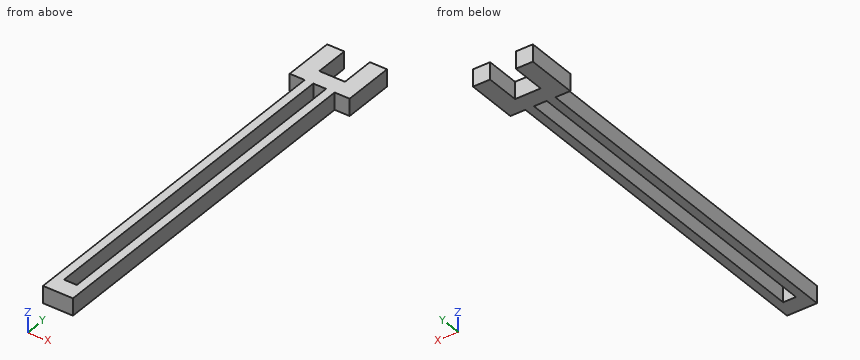
from build123d import *

# Parameters (mm, degrees)
F0_W     = 44.45
F0_H     = 25.4
F1_DEPTH = 533.4
F2_W     = 19.05
F2_H     = 508
F3_DEPTH = 25.4
F4_W     = 88.9
F4_H     = 25.4
F5_DEPTH = 76.2
F6_W     = 38.1
F6_H     = 50.8
F7_DEPTH = 25.4


with BuildPart() as f1:
    # F0 (on Front) → F1 (new body)
    with BuildSketch(Plane.XZ):
        Rectangle(F0_W, F0_H)
    extrude(amount=-F1_DEPTH)

    # F2 (on face) → F3 (cut)
    with BuildSketch(Plane.XY.offset(12.7)):
        with Locations((0, 279.4)):
            Rectangle(F2_W, F2_H)
    extrude(amount=-F3_DEPTH, mode=Mode.SUBTRACT)

    # F4 (on face) → F5 (join)
    with BuildSketch(Plane(origin=(0, 533.4, 0), x_dir=(-1, 0, 0), z_dir=(0, 1, 0))):
        Rectangle(F4_W, F4_H)
    extrude(amount=F5_DEPTH)

    # F6 (on face) → F7 (cut)
    with BuildSketch(Plane.XY.offset(12.7)):
        with Locations((0, 584.2)):
            Rectangle(F6_W, F6_H)
    extrude(amount=-F7_DEPTH, mode=Mode.SUBTRACT)


solid = f1.part
Geometry check sheet. Reference: the model listing, model coordinates, mm. Round coordinates to 2 decimals unless told otherwise and drop trailing zeros. Loops run counter-clockwise (first coordinate to the right, second up) from the corner with the lowest first, then second, coordinate; pieces in that order, holes last. Notation, with made-up numbers: (51.25, 37.25) - (60.25, 37.25) arc R18 cw to (60.25, 65.25) - close; hole circle Ø11 at (-31.75, 15.5). An arc over 180 degrees is marked (long way). One line per question, with ' | ' between items. Start each with the question number.
1. Cross-section at A-A on y = 262. Record the cut outline in (x, z) (3 decimals), then the cut area to 3 significant figures.
2. Cross-section at C-C on z = 2.25. Record the cut outline in (x, y) (3 decimals), then the cut area to 3 significant figures.
3. Scan lines: line 1 (X direction, y = 325, z = 8.75) (3 decimals); line 2 (X direction, y = 559, z = -11); line 3 (Y direction, x = 3, z = -3.75). Record each from-to range of solid material in increasing order. Write a range as [from, to].
4. Cross-section at D-D on x = 27.5. Record the cut outline in (y, z).
5. Cross-section at B-B on x = 4. Record the cut outline in (y, z), then the cut area to 3 significant figures.
6. Depth check by flat-ended pin: pin 1 (7.5 mm diameter, centred on y = 239.5, z = 5.5, fed in from +X) (3 decimals); pin 2 (11 mm diameter, centred on x = -29.5, z = -2.5, fed in from -Y); pin 3 (15 mm diameter, centred on x = 0, z = 2, fed in from +Y). Enter the tip coordinate at first touch or a pass-through.
Taken from the geometry:
1) outline: (-22.225, -12.7) - (-9.525, -12.7) - (-9.525, 12.7) - (-22.225, 12.7) - close; (9.525, -12.7) - (22.225, -12.7) - (22.225, 12.7) - (9.525, 12.7) - close | area: 645 mm²
2) outline: (-44.45, 533.4) - (-22.225, 533.4) - (-22.225, 0) - (22.225, 0) - (22.225, 533.4) - (44.45, 533.4) - (44.45, 609.6) - (19.05, 609.6) - (19.05, 558.8) - (-19.05, 558.8) - (-19.05, 609.6) - (-44.45, 609.6) - close; hole (-9.525, 25.4) - (9.525, 25.4) - (9.525, 533.4) - (-9.525, 533.4) - close | area: 18,900 mm²
3) line 1: [-22.225, -9.525], [9.525, 22.225] | line 2: [-44.45, -19.05], [19.05, 44.45] | line 3: [0, 25.4], [533.4, 558.8]
4) outline: (533.4, -12.7) - (609.6, -12.7) - (609.6, 12.7) - (533.4, 12.7) - close
5) outline: (0, -12.7) - (25.4, -12.7) - (25.4, 12.7) - (0, 12.7) - close; (533.4, -12.7) - (558.8, -12.7) - (558.8, 12.7) - (533.4, 12.7) - close | area: 1,290 mm²
6) pin 1: x = 22.225 | pin 2: y = 533.4 | pin 3: y = 558.8
